Geometry: final body of the model. Coordinates: model frame, mm. Face numbers are marked on the shaded views. Give positions to 0.01 mm unless a question says otherwise; leave off trailing zeros. Order: outer loops, then holes, each group sorted by start corner. A loop starts at its lowest first (then second) coordinate and runs counter-clockwise, first axis right, second up. Notation, with made-up numbers: (-0.75, 87) - (47.25, 87) arc R31 cw to (47.25, 113) - close; hole circle Ø6 at (89, 88.5). An arc over 180 degrees is marked (long way). Use one line per item in the form item = value.
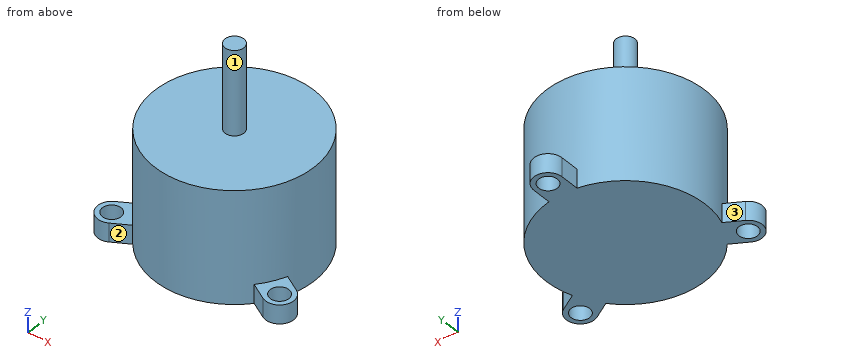
Autodesk Inventor part; units mm, degrees
ref_plane "YZ Plane" through (0, 0, 0) normal (1, 0, 0) x (0, 1, 0)
ref_plane "XZ Plane" through (0, 0, 0) normal (0, 1, 0) x (-1, 0, 0)
ref_plane "XY Plane" through (0, 0, 0) normal (0, 0, 1) x (1, 0, 0)
sketch "Sketch1" plane through (0, 0, 0) normal (0, 0, 1) x (1, 0, 0)
  circle A0 centre (0, 0) radius 8.5
  dimension "d0" = 17
extrude "Extrusion1" add sketch "Sketch1" along normal blind 12
sketch "Sketch2" plane through (0, 0, 0) normal (0, 0, -1) x (-1, 0, 0)
  circle A0 centre (0, 0) radius 8.5
  line L0 (-1.5, 8.3666) -> (-1.5, 10.3666)
  line L1 (1.5, 8.3666) -> (1.5, 10.3666)
  arc A1 (1.5, 10.3666) -> (-1.5, 10.3666) centre (0, 10.3666) ccw
  line L2 (-6.4957, -5.4823) -> (-8.2277, -6.4823)
  line L3 (-7.9957, -2.8843) -> (-9.7277, -3.8843)
  arc A2 (-9.7277, -3.8843) -> (-8.2277, -6.4823) centre (-8.9777, -5.1833) ccw
  line L4 (7.9957, -2.8843) -> (9.7277, -3.8843)
  line L5 (6.4957, -5.4823) -> (8.2277, -6.4823)
  arc A3 (8.2277, -6.4823) -> (9.7277, -3.8843) centre (8.9777, -5.1833) ccw
  arc A4 (-7.9957, -2.8843) -> (-6.4957, -5.4823) centre (0, 0) ccw
  arc A5 (6.4957, -5.4823) -> (7.9957, -2.8843) centre (0, 0) ccw
  dimension "d4" = 2
  dimension "d7" = 360
  dimension "d21" = 1.5
extrude "Extrusion2" add sketch "Sketch2" against normal blind 2 contours A0 L0 A1 L1 | L4 A3 L5 A0 | A0 L2 A2 L3
hole "Hole1" at (-8.9777, -5.1833, 0) at (8.9777, -5.1833, 0) at (0, 10.3666, 0) direction (0, 0, 1) diameter 2 end through all
sketch "Sketch3" plane through (0, 0, 12) normal (0, 0, 1) x (1, 0, 0)
  circle A0 centre (0, 0) radius 1
  dimension "d18" = 2
extrude "Extrusion3" add sketch "Sketch3" along normal blind 9
properties part number "motor_design2" material "Aluminum 6061-AHC"
(1) Contact query for flat-ended pins moving along their axis: pin 1 Ø10 at (x, z) = (2.5, 15) entering from -Y; pin 2 Ø3 at (y, z) = (-4.5, 4) entering from -X; pin 3 Ø1.1 at (x, y) = (-9, -4) entering from +Z; pin 4 Ø3.5 at (x, y) = (-0.5, 10) entering from +Z. Output: stop coordinate, or through.
Computed values:
pin_1 = -8.5
pin_2 = -7.95
pin_3 = 2
pin_4 = 12
(2) Cut plane D-D on z = 14.75. Output: boundary loops of the cut face in (x, y), plus the area to 3 significant figures.
Computed values:
outline = circle Ø2 at (0, 0)
area = 3.14 mm²
(3) Pull-direction query (X, two-part tool) for the marked faces 1, 2 and 3; classes: released by +X, released by -X, zero draft, split by the parting line, or undercut.
Computed values:
face_1 = split by the parting line
face_2 = undercut
face_3 = released by -X
(4) Cut plane A-A on x = 0. Output: boundary loops of the cut face in (y, z), plus the area to 3 significant figures.
Computed values:
outline = (-8.5, 0) - (9.37, 0) - (9.37, 2) - (8.5, 2) - (8.5, 12) - (1, 12) - (1, 21) - (-1, 21) - (-1, 12) - (-8.5, 12) - close; (11.37, 0) - (11.87, 0) - (11.87, 2) - (11.37, 2) - close
area = 225 mm²
(5) Cut plane B-B on y = 0. Output: boundary loops of the cut face in (x, z).
Computed values:
outline = (-8.5, 0) - (8.5, 0) - (8.5, 12) - (1, 12) - (1, 21) - (-1, 21) - (-1, 12) - (-8.5, 12) - close
(6) Cut plane C-C on y = 10. Output: boundary loops of the cut face in (x, z).
Computed values:
outline = (-1.5, 0) - (-0.93, 0) - (-0.93, 2) - (-1.5, 2) - close; (0.93, 0) - (1.5, 0) - (1.5, 2) - (0.93, 2) - close
(7) Ray query, line 1 along Z through (x, y) = (-1.5, 3); line 2 along Z through (x, y) = (8, -4.75); line 3 along Y through (x, z) = (-7.5, 2.75). Return the intervals inside material, ascending.
Computed values:
line_1 = 0 to 12
line_2 = 0 to 2
line_3 = -4 to 4
